Here's how the part is built. I have some questions about the finished solid (model axes, mm). Face numbers are marked on the shaded views. Give positions to 0.01 mm unless a question says otherwise; leave off trailing zeros. Write each loop counter-clockwise with the first axis right and the second up, starting at its lowest first coordinate (ties: lowest second). Pieces come first, ordered by that corner, then holes. Notation, with made-up numbers: (59, 61.25) -> (98, 61.25) arc R14 cw to (98, 82.25) -> close; hole circle Ø6 at (-31.5, -20.5). An arc over 180 degrees is marked (long way). Answer as CSV lines item,"result". Start each with the question number.
from build123d import *

# Parameters (mm, degrees)
ESBO_O1_R                = 5
RESSALTO_EXTRUS_O1_DEPTH = 10


with BuildPart() as part:
    # Esboço1 → Ressalto-extrusão1 (new body)
    with BuildSketch(Plane.XY):
        with BuildLine():
            Line((-27.286144523, -18.629908028), (-27.286144523, -28.629908028))
            Line((-27.286144523, -28.629908028), (27.286144523, -28.629908028))
            Line((27.286144523, -28.629908028), (27.286144523, -18.629908028))
            ThreePointArc((27.286144523, -18.629908028), (19.069349751, -10.682542862), (15, 0))
            ThreePointArc((15, 0), (0, 15), (-15, 0))
            ThreePointArc((-15, 0), (-19.069349751, -10.682542862), (-27.286144523, -18.629908028))
        make_face()
        Circle(ESBO_O1_R, mode=Mode.SUBTRACT)
    extrude(amount=RESSALTO_EXTRUS_O1_DEPTH)


solid = part.part
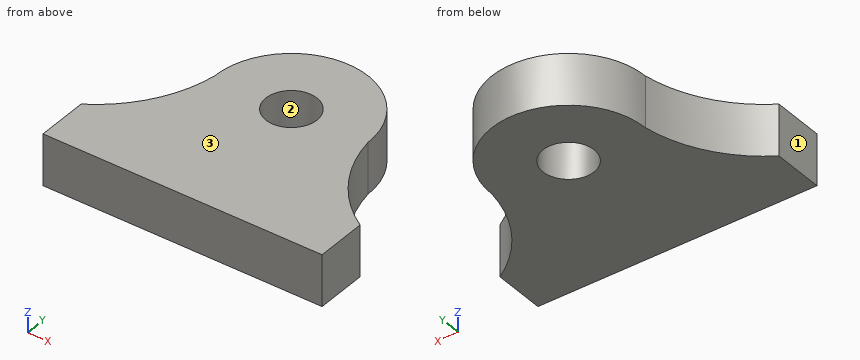
Item 1: If we section it at C-C (y = -2): Please give me the cut outline in (x, z), and give its area (3 significant figures).
Item 2: If we section it at D-D (x = 9): Please give me the cut outline in (y, z).
Item 3: If we section it at B-B (z = 6.75): Please give me the cut outline in (x, y).
Item 4: I'm going to push flat-ended pins straight in: pin 1 (4 mm diameter, centred on x = -19.5, z = 9, fed in from +Y); pin 2 (2 mm diameter, centred on x = 3.5, z = 7.5, fed in from +Y); pin 3 (2 mm diameter, centred on x = -21.5, z = 6.5, fed in from +Y). Where does each tip first touch, or does it pass through?
Item 5: If we section it at A-A (x = 0): Please give me the cut outline in (y, z), and give its area (3 significant figures).
Item 6: If I drill on line 1 (Y direction, x = 0, z = 2); line 2 (X direction, y = -4.5, z = 2); line 3 (Y direction, x = 12.5, z = 6.25), over which ranges is the centre line in solid material (lowest first)? Write a range as [from, to].
Item 7: We'd pull the mould along X, two halves only. Please class the marked faces 1, 2 and 3: released by +X, released by -X, zero draft, split by the parting line, or undercut.
Final values:
1,outline,"(-15.37, 0) -> (-4.58, 0) -> (-4.58, 10) -> (-15.37, 10) -> close; (4.58, 0) -> (15.37, 0) -> (15.37, 10) -> (4.58, 10) -> close"
1,area,"216 mm2"
2,outline,"(-28.63, 0) -> (12, 0) -> (12, 10) -> (-28.63, 10) -> close"
3,outline,"(-27.29, -28.63) -> (27.29, -28.63) -> (27.29, -18.63) arc R26.3 cw to (15, 0) arc R15 ccw to (-15, 0) arc R26.3 cw to (-27.29, -18.63) -> close; hole circle Ø10 at (0, 0)"
4,pin 1,"y = -7.96"
4,pin 2,"y = 14.79"
4,pin 3,"y = -12.65"
5,outline,"(-28.63, 0) -> (-5, 0) -> (-5, 10) -> (-28.63, 10) -> close; (5, 0) -> (15, 0) -> (15, 10) -> (5, 10) -> close"
5,area,"336 mm2"
6,line 1,"[-28.63, -5], [5, 15]"
6,line 2,"[-16.07, -2.18], [2.18, 16.07]"
6,line 3,"[-28.63, 8.29]"
7,face 1,"released by -X"
7,face 2,"undercut"
7,face 3,"zero draft"
